Input: part model. Units: mm. Frame: model coordinates. Face numbers are marked on the shaded views. A direction names the side the tool comes from. Coordinates: 2 decimals unless noted, no trailing zeros. Write each loop counter-clockwise with the first axis right and the second up, starting at its lowest first coordinate (ties: lowest second). Pieces come first, ordered by that corner, then holes. Notation, with made-up numbers: (46, 8) - (104, 8) arc R32 cw to (104, 45) - close; hole circle Ø1 at (7, 43). An arc over 180 degrees is marked (long way). One line per question, with ' | ' between items. Start each with the question number.
1) First-contact query: P1, Ø1, axis at x = -3, z = -2.5, coming from the +Y side; P2, Ø4, axis at x = -5.5, y = 4.5, coming from the +Z side; P3, Ø3, axis at x = 8.65, z = 0, coming from the -Y side. Flat tips, straight axial feed; report the tip coordinate or a pass-through.
2) Section query D-D on x = 0.75. Return loops of the section in (y, z).
3) Reachability of the marked faces 1, 2 and 3 from +Z, -Z, +X, -X, +Y, -Y: full face, straight path, thin tool, end or side. Return the list, or none.
4) Section query B-B on z = 0. Return loops of the section in (x, y).
5) Section query A-A on y = 4. Return loops of the section in (x, z).
6) Line query: line 1 (X direction, y = 0.55, z = 0); line 2 (Z direction, x = 2.5, y = 4); line 3 (Y direction, x = -3, z = 1.5). Output: solid intervals per line, ascending.
7) Section query C-C on z = -9. Return loops of the section in (x, y), and give its area (3 significant figures).
```python
from build123d import *

# Parameters (mm, degrees)
SKETCH_1_W      = 30
SKETCH_1_H      = 15
SKETCH_1_R      = 1.75
EXTRUDE_1_DEPTH = 1.5
FILLET_1_R      = 5
EXTRUDE_3_DEPTH = 5


with BuildPart() as part:
    # 草图1 → 凸台-拉伸1 (new body)
    with BuildSketch(Plane(origin=(0, 0, 0), x_dir=(1, 0, 0), z_dir=(0, 1, 0))):
        Rectangle(SKETCH_1_W, SKETCH_1_H)
        with Locations(Location((-8.867330988, 0, 0), (0, 0, 270))):
            Circle(SKETCH_1_R, mode=Mode.SUBTRACT)
        with Locations(Location((8.647397187, 0, 0), (0, 0, 270))):
            Circle(SKETCH_1_R, mode=Mode.SUBTRACT)
    extrude(amount=EXTRUDE_1_DEPTH)

    # 圆角1
    fillet_1_edges = [part.edges().sort_by_distance(p)[0] for p in [
        (15, 0.75, 7.5),
        (-15, 0.75, 7.5),
    ]]
    fillet(fillet_1_edges, radius=FILLET_1_R)

    # 草图2 → 凸台-拉伸3 (add, symmetric)
    with BuildSketch(Plane(origin=(0, 0, 0), x_dir=(0, 0, -1), z_dir=(1, 0, 0))):
        with BuildLine():
            Line((4.938262309, 2.520980054), (4.5, 2.267949192))
            ThreePointArc((4.5, 2.267949192), (4.086336582, 2.228506303), (3.785714286, 2.515385022))
            ThreePointArc((3.785714286, 2.515385022), (9.742937815, 7.311982783), (7.5, 0))
            Line((7.5, 0), (7.5, 1.5))
            ThreePointArc((7.5, 1.5), (8.926677651, 6.052946877), (5.156885257, 3.128327297))
            ThreePointArc((5.156885257, 3.128327297), (5.15871146, 2.784648148), (4.938262309, 2.520980054))
        make_face()
    extrude(amount=EXTRUDE_3_DEPTH, both=True)


solid = part.part
```
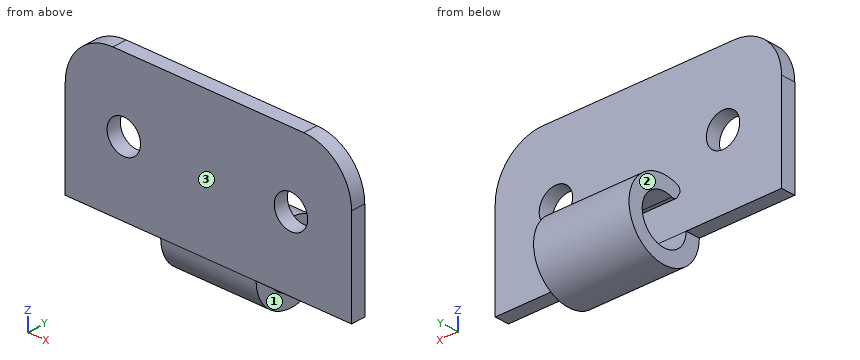
Answer key:
1) P1: y = 1.5 | P2: z = -3.5 | P3: through
2) outline: (0, -7.5) arc R4 ccw (long way) to (2.52, -3.79) arc R0.5 ccw to (2.27, -4.5) - (2.52, -4.94) arc R0.5 ccw to (3.13, -5.16) arc R2.5 cw (long way) to (1.5, -7.5) - (1.5, 7.5) - (0, 7.5) - close
3) face 1: -Z, +X, +Y | face 2: -Z, -X, +Y | face 3: +Z, -Z, +X, -X, -Y
4) outline: (-15, 0) - (-10.62, 0) - (-10.62, 1.5) - (-15, 1.5) - close; (-7.12, 0) - (6.9, 0) - (6.9, 1.5) - (-7.12, 1.5) - close; (10.4, 0) - (15, 0) - (15, 1.5) - (10.4, 1.5) - close
5) outline: (-5, -11.5) - (5, -11.5) - (5, -10) - (-5, -10) - close; (-5, -5) - (5, -5) - (5, -3.5) - (-5, -3.5) - close
6) line 1: -15 to -10.62, -7.12 to 6.9, 10.4 to 15 | line 2: -11.5 to -10, -5 to -3.5 | line 3: 0 to 1.5
7) outline: (-5, 0.29) - (5, 0.29) - (5, 2) - (-5, 2) - close; (-5, 6) - (5, 6) - (5, 7.71) - (-5, 7.71) - close | area: 34.2 mm²
